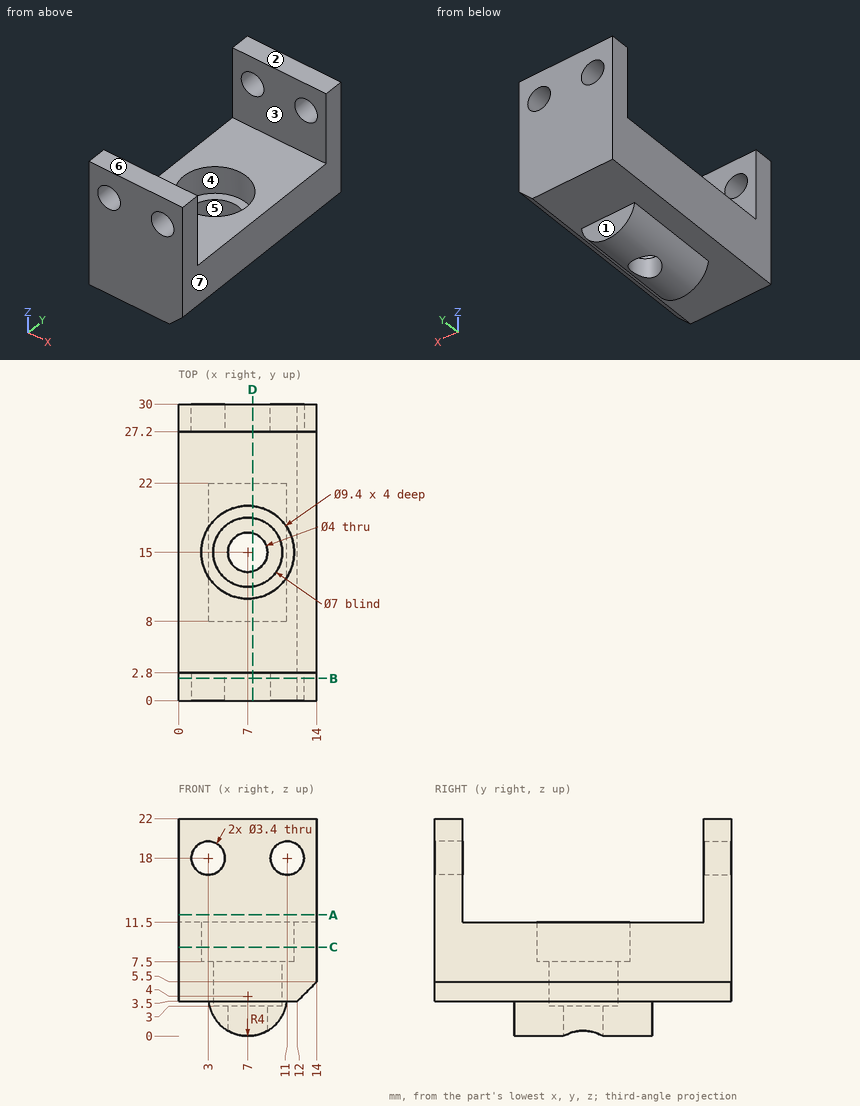
Answer from the drawing. Dimensions are ordinates in mm from the lowest x, y and z of the part. A direction names the side the tool comes from. Give positions to 0.01 mm unless a question says otherwise; leave off trailing zeros. Write each loop counter-clockwise with the first axis right and the second up, starting at its lowest first coordinate (ties: lowest second). Pieces come first, ordered by that corner, then holes. Notation, with made-up numbers: (10.5, 75) -> (53.5, 75) arc R20 cw to (53.5, 81) -> close; hole circle Ø4 at (76.5, -39). An arc over 180 degrees is marked (long way). Use a Markdown table: item, result.
(1) Section D-D, the plane x = 7.5 is taken. Determine the outline of the cut face in (y, z).
Return value:
| item | result |
|---|---|
| outline | (0, 3.5) -> (8, 3.5) -> (8, 0.03) -> (13.06, 0.03) -> (13.06, 3) -> (11.54, 3) -> (11.54, 7.5) -> (10.33, 7.5) -> (10.33, 11.5) -> (2.8, 11.5) -> (2.8, 22) -> (0, 22) -> close; (16.94, 0.03) -> (22, 0.03) -> (22, 3.5) -> (30, 3.5) -> (30, 22) -> (27.2, 22) -> (27.2, 11.5) -> (19.67, 11.5) -> (19.67, 7.5) -> (18.46, 7.5) -> (18.46, 3) -> (16.94, 3) -> close |
(2) Flat-ended cylindrical pins translate along their axes: P1, Ø1, axis at x = 9, y = 23, coming from the +Z side; P2, Ø5.5, axis at x = 7, y = 15, coming from the +Z side; P3, Ø4.5, axis at x = 8, y = 16, coming from the +Z side. Find the tip coordinate at first contact, or state that the pin passes through.
Return value:
| item | result |
|---|---|
| P1 | z = 11.5 |
| P2 | z = 3 |
| P3 | z = 7.5 |
(3) Determine the mould class of the marked faces 5, 6 and 7 for opening direction X: released by +X, released by -X, zero draft, split by the parting line, or undercut.
Return value:
| item | result |
|---|---|
| face 5 | undercut |
| face 6 | zero draft |
| face 7 | released by +X |
(4) Section C-C, the plane z = 9 is taken. Determine the outline of the cut face in (x, y).
Return value:
| item | result |
|---|---|
| outline | (0, 0) -> (14, 0) -> (14, 30) -> (0, 30) -> close; hole circle Ø9.4 at (7, 15) |
(5) Find the intervals of material crossed by probe 1 along Z at (x, y) = (11, 28.3); probe 2 along Y at (x, z) = (1.5, 16.75); probe 3 along Y at (x, z) = (7, 5.95), in increasing order. Write a range as from..to.
Return value:
| item | result |
|---|---|
| probe 1 | 3.5..16.3, 19.7..22 |
| probe 2 | 0..2.8, 27.2..30 |
| probe 3 | 0..11.5, 18.5..30 |
(6) For the marked faces 1, 2, 3 and 4, determine the directions among +Z, -Z, +X, -X, +Y, -Y from which every point of the face is accessible in a straight line to the end or side of a thin tool.
Return value:
| item | result |
|---|---|
| face 1 | -Z, +X, -X, +Y |
| face 2 | +Z, +X, -X, +Y, -Y |
| face 3 | +Z, +X, -X |
| face 4 | +Z |
(7) Section A-A, the plane z = 12.25 is taken. Determine the outline of the cut face in (x, y).
Return value:
| item | result |
|---|---|
| outline | (0, 0) -> (14, 0) -> (14, 2.8) -> (0, 2.8) -> close; (0, 27.2) -> (14, 27.2) -> (14, 30) -> (0, 30) -> close |
(8) Section B-B, the plane y = 2.25 is taken. Determine the outline of the cut face in (x, z), then the cut area to 3 significant figures.
Return value:
| item | result |
|---|---|
| outline | (0, 3.5) -> (12, 3.5) -> (14, 5.5) -> (14, 22) -> (0, 22) -> close; hole circle Ø3.4 at (3, 18); hole circle Ø3.4 at (11, 18) |
| area | 239 mm2 |
